Can you work these out from the model? Positions are in its coordinate system, mm. Face numbers are marked on the shaded views. A direction names the side the tool comes from. Give positions to 0.01 mm unless a question says otherwise; leave off trailing zeros. Loops run counter-clockwise (first coordinate to the right, second up) from the corner with the lowest first, then second, coordinate; pieces in that order, holes last. Notation, with made-up numbers: (-38.75, -38.75) -> (-20.75, -38.75) arc R27 cw to (-20.75, -8.75) -> close; hole circle Ø10 at (31.5, 21.25). An arc over 180 degrees is marked (long way). Return JSON: item names as keys, results as strings. Group by question number.
Q1. Suppose I cut it at A-A, the plane x = -4.25. Please give me the cut outline in (y, z).
Q2. I need wall thicknesses on line 1 along Y through (x, z) = (3.7, 0); line 2 along Y through (x, z) = (-3.25, 2); line 3 along X through (y, z) = (-2.5, 5.75). Which ranges of each line are inside material? Lowest first, please. Write a range as [from, to].
Q3. Which directions (+Z, -Z, +X, -X, +Y, -Y) give clear straight access to the entire face, cutting with the end or side of a thin tool? Please do the marked faces 1, 2, 3, 4 and 5.
Q4. Will these pins go through, and if not, where does the flat tip stop? pin 1 (1.9 mm diameter, centred on y = 0.5, z = -0.5, fed in from -X); pin 2 (5 mm diameter, centred on x = 2, y = -4, fed in from -Z).
Q5. Thinking about a two-plate mould opening in Y: for the marked faces 6, 7, 8 and 9, which applies, pulls with the +Y half, pulls with the -Y half, needs draft (parallel to the pull), parting line crosses it, or undercut?
```python
from build123d import *

# Parameters (mm, degrees)
SKETCH1_R           = 6.35
BOSS_EXTRUDE1_DEPTH = 1.5875
SKETCH2_R           = 4.826
SKETCH2_R_2         = 3.2385
BOSS_EXTRUDE2_DEPTH = 6.2865
CHAMFER1_SIZE       = 0.381
FILLET2_R           = 0.635


with BuildPart() as part:
    # Sketch1 → Boss-Extrude1 (new body, symmetric)
    with BuildSketch(Plane(origin=(0, 0, 0), x_dir=(0, 0, -1), z_dir=(1, 0, 0))):
        Circle(SKETCH1_R)
    extrude(amount=BOSS_EXTRUDE1_DEPTH, both=True)

    # Sketch2 → Boss-Extrude2 (add, symmetric)
    with BuildSketch(Plane(origin=(0, 0, 0), x_dir=(0, 0, -1), z_dir=(1, 0, 0))):
        Circle(SKETCH2_R)
        Circle(SKETCH2_R_2, mode=Mode.SUBTRACT)
    extrude(amount=BOSS_EXTRUDE2_DEPTH, both=True)

    # Chamfer1
    chamfer1_edges = [part.edges().sort_by_distance(p)[0] for p in [
        (-6.2865, 0, 4.826),
        (6.2865, 0, 4.826),
        (-6.2865, 0, 3.2385),
        (6.2865, 0, 3.2385),
    ]]
    chamfer(chamfer1_edges, length=CHAMFER1_SIZE)

    # Fillet2
    fillet2_edges = [part.edges().sort_by_distance(p)[0] for p in [
        (-1.5875, 0, 4.826),
        (1.5875, 0, 4.826),
    ]]
    fillet(fillet2_edges, radius=FILLET2_R)

    # Cut-Sweep1: sweep along a path in Sketch3
    with BuildLine(Plane(origin=(0, 0, 0), x_dir=(0, 0, -1), z_dir=(1, 0, 0))) as cut_sweep1_path:
        CenterArc((0, 0), 6.35, 0, 360)
    # Sketch7 → Cut-Sweep1 (sweep, cut)
    with BuildSketch(Plane(origin=(0, 0, 0), x_dir=(1, 0, 0), z_dir=(0, 1, 0))):
        Polygon((1.27, -6.764445418), (-1.27, -6.764445418), (0, -5.494445418), align=None)
    sweep(path=cut_sweep1_path.line, mode=Mode.SUBTRACT)


solid = part.part
```
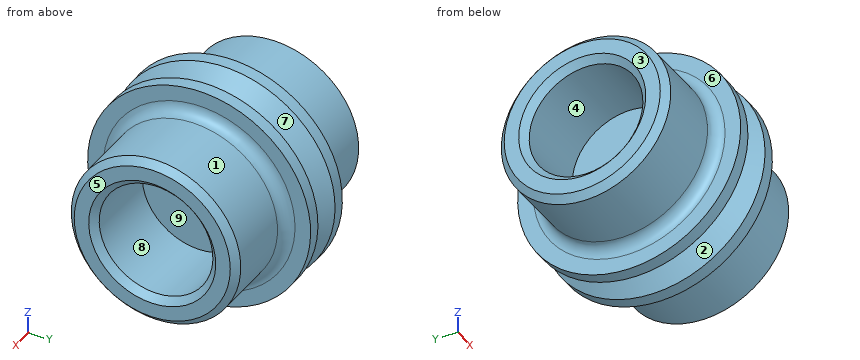
Ans:
{
 "1": {"outline": "circle Ø9.65 at (0, 0); hole circle Ø6.48 at (0, 0)"},
 "2": {"line 1": "y = [-4.83, -3.24], [3.24, 4.83]", "line 2": "y = [-4.39, -2.55], [2.55, 4.39]", "line 3": "x = [-1.59, -0.78], [0.78, 1.59]"},
 "3": {"face 1": "+X", "face 2": "none", "face 3": "+Z, -Z, -X, +Y, -Y", "face 4": "-X", "face 5": "+Z, -Z, +X, +Y, -Y"},
 "4": {"pin 1": "stops at x = -1.59", "pin 2": "stops at z = -6.16"},
 "5": {"face 6": "needs draft", "face 7": "parting line crosses it", "face 8": "undercut", "face 9": "undercut"}
}
